Build history of the part. All positions in model axes, mm. A direction names the side the tool comes from. Give positions to 0.01 mm unless a question says otherwise; leave off trailing zeros. Order: outer loops, then holes, each group sorted by start corner. A loop starts at its lowest first (then second) coordinate and runs counter-clockwise, first axis right, second up. Notation, with made-up numbers: (-26.5, -10.5) - (-19.5, -10.5) arc R18 ccw to (-19.5, 0.5) - close; hole circle Ø11 at (-11.5, -27). An arc over 180 degrees is marked (long way). Use a Markdown table: item, result. Add a question column.
(1) Mould opens along X. For faces 1 (the face through (25.427, 4.93, 53.002)), 2 (the face through (0, 5, 114)), 3 (the face through (0, 5, 140)) say: +X half, -X half, draft (parallel to the pull), parting line (faces both ways), or undercut.
(2) Flat gauge pins, fed straight in: pin 1 (2 mm diameter, centred on y = 6.5, z = 123.5, fed in from +X); pin 2 (10 mm diameter, centred on x = 0, z = 24, fed in from +Y); pin 3 (4 mm diameter, centred on y = 6.5, z = 103, fed in from +X); pin 4 (4 mm diameter, centred on y = 7.5, z = 117, fed in from -X). Where does each tip first touch, or does it go through?
(3) Which spindle directions (+Z, -Z, +X, -X, +Y, -Y) get a long thin tool onto all of the face, cutting with end or side? Do faces 4 (the face through (-12.5, 5, 117)), 5 (the face through (6.5, 5, 124)), 6 (the face through (12.5, 5, 117)). Say none if no direction does.
(4) Wall check: line 1 (Z direction, x = 0, y = 2.15); line 2 (X direction, y = 7, z = 125.5); line 3 (Z direction, x = 3, y = 5.75). Give the ranges that are in metal, low to high.
(5) Slice it at D-D (z = 109.5). Write the cut outline in (x, y).
(6) Slice it at C-C (z = -24). Write the cut outline in (x, y), then the cut area to 3 significant figures.
(7) Slice it at A-A (x = 0). Write the cut outline in (y, z).
(8) Slice it at B-B (y = 7.75). Write the cut outline in (x, z).
Autodesk Inventor part; units mm, degrees
ref_plane "YZ Plane" through (0, 0, 0) normal (1, 0, 0) x (0, 1, 0)
ref_plane "XZ Plane" through (0, 0, 0) normal (0, 1, 0) x (-1, 0, 0)
ref_plane "XY Plane" through (0, 0, 0) normal (0, 0, 1) x (1, 0, 0)
sketch "Эскиз1" plane through (0, 0, 0) normal (0, 1, 0) x (-1, 0, 0)
  arc A0 (-38, 0) -> (38, 0) centre (0, 0) ccw
  line L0 (53.2, 0) -> (-53.2, 0)
  line L1 (38, 0) -> (12.5, 107.5)
  line L2 (-38, 0) -> (-12.5, 107.5)
  line L3 (-12.5, 107.5) -> (-12.5, 127.5)
  line L4 (12.5, 107.5) -> (12.5, 127.5)
  arc A1 (12.5, 127.5) -> (-12.5, 127.5) centre (0, 127.5) ccw
  line L5 (0, -73.6) -> (0, 175.6)
  line L6 (6.5, 120.5) -> (6.5, 127.5)
  line L7 (-6.5, 120.5) -> (-6.5, 127.5)
  arc A2 (-6.5, 120.5) -> (6.5, 120.5) centre (0, 120.5) ccw
  arc A3 (6.5, 127.5) -> (-6.5, 127.5) centre (0, 127.5) ccw
  dimension "d1" = 76
  dimension "d2" = 25
  dimension "d3" = 20
  dimension "d4" = 127.5
  dimension "d5" = 7
  dimension "d6" = 13
extrude "Выдавливание1" add sketch "Эскиз1" along normal blind 10 contours L0 L5 A0 | L2 L3 A1 L5 A3 L7 A2 L0 | L5 L0 A0 | L5 A2 L6 A3 A1 L4 L1 L0
sketch "Эскиз2" plane through (0, 10, 0) normal (0, 1, 0) x (1, 0, 0)
  point P0 (0, 0)
  point P1 (0, 24)
  point P2 (0, -24)
  dimension "d9" = 24
  dimension "d10" = 48
hole "Отверстие1" at (0, 10, -24) at (0, 10, 24) direction (0, -1, 0) diameter 11 end through all countersink diameter 20.4 countersink angle 90
fillet "Сопряжение1" radius 2 4 edges at (12.5, 5, 107.5) (38, 5, 0) (-12.5, 5, 107.5) (-38, 5, 0)
properties part number "Рычаг"
Solution:
| question | item | result |
|---|---|---|
| 1 | face 1 | +X half |
| 1 | face 2 | undercut |
| 1 | face 3 | parting line |
| 2 | pin 1 | x = 12.5 |
| 2 | pin 2 | through |
| 2 | pin 3 | x = 14.04 |
| 2 | pin 4 | x = -12.5 |
| 3 | face 4 | +Z, -X, +Y, -Y |
| 3 | face 5 | +Y, -Y |
| 3 | face 6 | +Z, +X, +Y, -Y |
| 4 | line 1 | -38 to -29.5, -18.5 to 18.5, 29.5 to 114, 134 to 140 |
| 4 | line 2 | -12.5 to -6.5, 6.5 to 12.5 |
| 4 | line 3 | -37.88 to -29.14, -18.86 to 18.86, 29.14 to 114.73, 133.27 to 139.63 |
| 5 | outline | (-12.5, 0) - (12.5, 0) - (12.5, 10) - (-12.5, 10) - close |
| 6 | outline | (-29.46, 0) - (-5.5, 0) - (-5.5, 5.3) - (-10.2, 10) - (-29.46, 10) - close; (5.5, 0) - (29.46, 0) - (29.46, 10) - (10.2, 10) - (5.5, 5.3) - close |
| 6 | area | 457 mm2 |
| 7 | outline | (0, -38) - (10, -38) - (10, -34.2) - (5.3, -29.5) - (0, -29.5) - close; (0, -18.5) - (5.3, -18.5) - (10, -13.8) - (10, 13.8) - (5.3, 18.5) - (0, 18.5) - close; (0, 29.5) - (5.3, 29.5) - (10, 34.2) - (10, 114) - (0, 114) - close; (0, 134) - (10, 134) - (10, 140) - (0, 140) - close |
| 8 | outline | (-38, -0.24) arc R38 ccw to (38, -0.24) arc R2 ccw to (37.95, 0.23) - (12.55, 107.27) arc R2 cw to (12.5, 107.73) - (12.5, 127.5) arc R12.5 ccw to (-12.5, 127.5) - (-12.5, 107.73) arc R2 cw to (-12.55, 107.27) - (-37.95, 0.23) arc R2 ccw to start; hole circle Ø15.9 at (0, -24); hole circle Ø15.9 at (0, 24); hole (-6.5, 120.5) arc R6.5 ccw to (6.5, 120.5) - (6.5, 127.5) arc R6.5 ccw to (-6.5, 127.5) - close |
